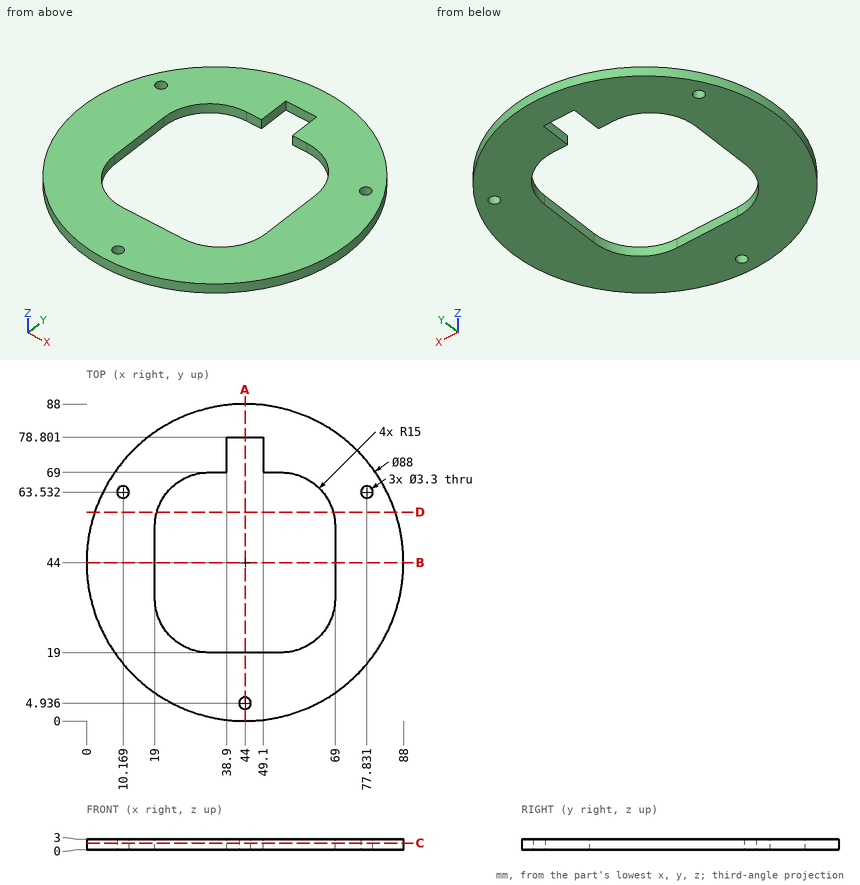
Verification items for this drawing (mm, ordinates from the low corner). Round coordinates to 2 decimals unless told otherwise and drop trailing zeros. Write each loop counter-clockwise with the first axis right and the second up, starting at its lowest first coordinate (ties: lowest second). Pieces come first, ordered by that corner, then holes. Notation, with made-up numbers: (50, 9.5) - (54, 9.5) arc R23 ccw to (54, 34.5) - close; hole circle Ø4 at (-8.5, -11.75). An arc over 180 degrees is marked (long way). Answer as a JSON object with one key per item and string values. Group by question number.
Q1. Section check A-A, the plane x = 44. Enter the section's corners in (y, z) (1 decimal).
Q2. Section check C-C, the plane z = 1.85. Give the number of separate pieces and of enclosed holes in the cut face, plus the area to 3 significant figures.
Q3. Section check B-B, the plane y = 44. Enter the section's corners in (x, z).
Q4. Go/stop test with flat-tipped pins: pin 1 Ø0.9 at (x, z) = (50.5, 1.5) entering from -Y; pin 2 Ø1.5 at (y, z) = (42, 2) entering from +X; pin 3 Ø1.5 at (x, z) = (50, 1) entering from -Y; pin 4 Ø2 at (x, y) = (10.17, 63.53) entering from -Z. Record where each tip stops, or that it passes through.
Q5. Thickness scan on line 1 (Y direction, x = 44, z = 1.8) (1 decimal); line 2 (X direction, y = 38, z = 1.2); line 3 (X direction, y = 64.5, z = 1.9) (1 decimal). Record the ranges inside material, lowest first.
Q6. Section check D-D, the plane y = 58. Enter the section's corners in (x, z).
Found:
{
 "1": {"outline": "(0, 0) - (3.3, 0) - (3.3, 3) - (0, 3) - close; (6.6, 0) - (19, 0) - (19, 3) - (6.6, 3) - close; (78.8, 0) - (88, 0) - (88, 3) - (78.8, 3) - close"},
 "2": {"separate pieces": "1", "enclosed holes": "4", "area": "3,650 mm^2"},
 "3": {"outline": "(0, 0) - (19, 0) - (19, 3) - (0, 3) - close; (69, 0) - (88, 0) - (88, 3) - (69, 3) - close"},
 "4": {"pin 1": "stops at y = 0.42", "pin 2": "stops at x = 87.98", "pin 3": "stops at y = 0.31", "pin 4": "passes through"},
 "5": {"line 1": "y = 0 to 3.3, 6.6 to 19, 78.8 to 88", "line 2": "x = 0.41 to 19, 69 to 87.59", "line 3": "x = 5.1 to 8.8, 11.5 to 23.3, 64.7 to 76.5, 79.2 to 82.9"},
 "6": {"outline": "(2.29, 0) - (19.54, 0) - (19.54, 3) - (2.29, 3) - close; (68.46, 0) - (85.71, 0) - (85.71, 3) - (68.46, 3) - close"}
}
